```python
from build123d import *

# Parameters (mm, degrees)
SKETCH_W        = 20
SKETCH_H        = 20
PAD_DEPTH       = 6
SKETCH001_R     = 5.5
POCKET_DEPTH    = 3.6
SKETCH002_R     = 3.1
POCKET001_DEPTH = 5
SKETCH003_W     = 5.8
SKETCH003_H     = 5
PAD001_DEPTH    = 6
SKETCH004_W     = 5
SKETCH004_H     = 5.8
PAD002_DEPTH    = 6
SKETCH005_W     = 5.8
SKETCH005_H     = 5
PAD003_DEPTH    = 6
SKETCH006_W     = 5
SKETCH006_H     = 5.8
PAD004_DEPTH    = 6
FILLET_R        = 1.2
FILLET001_R     = 1.2
FILLET002_R     = 1.2
FILLET003_R     = 1.2
FILLET004_R     = 1
FILLET005_R     = 1
FILLET006_R     = 1
FILLET007_R     = 1
FILLET008_R     = 1
FILLET009_R     = 1
FILLET010_R     = 1
FILLET011_R     = 1


with BuildPart() as part:
    # Sketch → Pad (new body)
    with BuildSketch(Plane.XY):
        with Locations((10, 10)):
            Rectangle(SKETCH_W, SKETCH_H)
    extrude(amount=PAD_DEPTH)

    # Sketch001 → Pocket (cut)
    with BuildSketch(Plane.XY.offset(6)):
        with Locations((10, 10)):
            Circle(SKETCH001_R)
    extrude(amount=-POCKET_DEPTH, mode=Mode.SUBTRACT)

    # Sketch002 → Pocket001 (cut)
    with BuildSketch(Plane.XY.offset(2.4)):
        with Locations((10, 10)):
            Circle(SKETCH002_R)
    extrude(amount=-POCKET001_DEPTH, mode=Mode.SUBTRACT)

    # Sketch003 → Pad001 (new body)
    with BuildSketch(Plane(origin=(0, 0, 0), x_dir=(1, 0, 0), z_dir=(0, 0, -1))):
        with Locations((10, -2.5)):
            Rectangle(SKETCH003_W, SKETCH003_H)
    extrude(amount=PAD001_DEPTH)

    # Sketch004 → Pad002 (new body)
    with BuildSketch(Plane(origin=(0, 0, 0), x_dir=(1, 0, 0), z_dir=(0, 0, -1))):
        with Locations((17.5, -10)):
            Rectangle(SKETCH004_W, SKETCH004_H)
    extrude(amount=PAD002_DEPTH)

    # Sketch005 → Pad003 (new body)
    with BuildSketch(Plane(origin=(0, 0, 0), x_dir=(1, 0, 0), z_dir=(0, 0, -1))):
        with Locations((10, -17.5)):
            Rectangle(SKETCH005_W, SKETCH005_H)
    extrude(amount=PAD003_DEPTH)

    # Sketch006 → Pad004 (new body)
    with BuildSketch(Plane(origin=(0, 0, 0), x_dir=(1, 0, 0), z_dir=(0, 0, -1))):
        with Locations((2.5, -10)):
            Rectangle(SKETCH006_W, SKETCH006_H)
    extrude(amount=PAD004_DEPTH)

    # Fillet
    fillet_edges = [part.edges().sort_by_distance(p)[0] for p in [
        (10, 20, 6),
    ]]
    fillet(fillet_edges, radius=FILLET_R)

    # Fillet001
    fillet001_edges = [part.edges().sort_by_distance(p)[0] for p in [
        (10, 0, 6),
    ]]
    fillet(fillet001_edges, radius=FILLET001_R)

    # Fillet002
    fillet002_edges = [part.edges().sort_by_distance(p)[0] for p in [
        (0, 10, 6),
    ]]
    fillet(fillet002_edges, radius=FILLET002_R)

    # Fillet003
    fillet003_edges = [part.edges().sort_by_distance(p)[0] for p in [
        (20, 10, 6),
    ]]
    fillet(fillet003_edges, radius=FILLET003_R)

    # Fillet004
    fillet004_edges = [part.edges().sort_by_distance(p)[0] for p in [
        (15, 10, -6),
    ]]
    fillet(fillet004_edges, radius=FILLET004_R)

    # Fillet005
    fillet005_edges = [part.edges().sort_by_distance(p)[0] for p in [
        (10, 5, -6),
    ]]
    fillet(fillet005_edges, radius=FILLET005_R)

    # Fillet006
    fillet006_edges = [part.edges().sort_by_distance(p)[0] for p in [
        (10, 15, -6),
    ]]
    fillet(fillet006_edges, radius=FILLET006_R)

    # Fillet007
    fillet007_edges = [part.edges().sort_by_distance(p)[0] for p in [
        (5, 10, -6),
    ]]
    fillet(fillet007_edges, radius=FILLET007_R)

    # Fillet008
    fillet008_edges = [part.edges().sort_by_distance(p)[0] for p in [
        (20, 10, -6),
    ]]
    fillet(fillet008_edges, radius=FILLET008_R)

    # Fillet009
    fillet009_edges = [part.edges().sort_by_distance(p)[0] for p in [
        (10, 0, -6),
    ]]
    fillet(fillet009_edges, radius=FILLET009_R)

    # Fillet010
    fillet010_edges = [part.edges().sort_by_distance(p)[0] for p in [
        (10, 20, -6),
    ]]
    fillet(fillet010_edges, radius=FILLET010_R)

    # Fillet011
    fillet011_edges = [part.edges().sort_by_distance(p)[0] for p in [
        (0, 10, -6),
    ]]
    fillet(fillet011_edges, radius=FILLET011_R)


solid = part.part
```
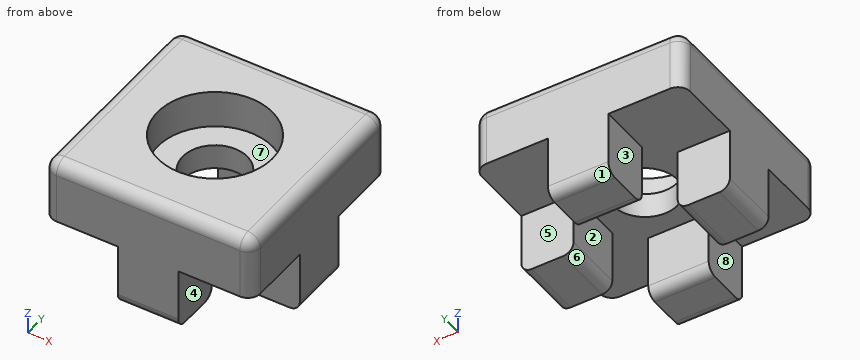
Here's how the part is built. I have some questions about the finished solid (model axes, mm). Face numbers are marked on the shaded views. A direction names the side the tool comes from. Give positions to 0.01 mm unless a question says otherwise; leave off trailing zeros. Order: outer loops, then holes, each group sorted by start corner. A loop starts at its lowest first (then second) coordinate and runs counter-clockwise, first axis right, second up. Notation, with made-up numbers: M -27,-37 L -10,-37 A16 cw -10,-9 Z; hole C -36,24.25 d2. An arc over 180 degrees is marked long. Use a Markdown table: item, result. Add a question column.
1. I need wall thicknesses on probe 1 along Y at (x, z) = (10, 1.3); probe 2 along Y at (x, z) = (10, 3.25); probe 3 along Z at (x, y) = (4.5, 5). Which ranges of each line are inside material? Lowest first, please. Write a range as from..to.
2. On a 3-axis mill with a long thin cutter (end or side, diameter ignored), from which of +Z, -Z, +X, -X, +Y, -Y can I reach the whole of each face in a straight line? I mean the marked faces 4, 5, 6, 7 and 8. Say none if no direction works.
3. Suppose I cut it at B-B (y = 16.25). List the corners of the cut face in (x, z) for me, and give its area (3 significant figures).
4. If we mould it in two halves opening along X, with no side actions, what happens to the marked faces 1, 2 and 3? For each: +X half, -X half, draft (parallel to the pull), parting line (faces both ways), or undercut.
5. Suppose I cut it at C-C (x = 10). List the corners of the cut face in (y, z) for me, and give its area (3 significant figures).
6. Suppose I cut it at D-D (z = -2.25). List the corners of the cut face in (x, y) for me.
7. Suppose I cut it at A-A (z = 4.25). List the corners of the cut face in (x, y) for me.
8. For pin 1 Ø1.5 at (y, z) = (16.5, -1.5) entering from -X; pin 2 Ø1.5 at (x, z) = (16.5, -3.5) entering from -Y; pin 3 Ø1.5 at (y, z) = (3, -2) entering from +X, each with a flat end and sliding along its axis, tell me the tip position at first contact or that it passes through.
Results list:
| question | item | result |
|---|---|---|
| 1 | probe 1 | y = 0..6.9, 13.1..20 |
| 1 | probe 2 | y = 0..4.5, 15.5..20 |
| 1 | probe 3 | z = 0..6 |
| 2 | face 4 | -Z, +X, +Y, -Y |
| 2 | face 5 | -Z, +X, -X, +Y |
| 2 | face 6 | -Z, +Y, -Y |
| 2 | face 7 | +Z |
| 2 | face 8 | -Z, -X, +Y, -Y |
| 3 | outline | M 0,0 L 7.1,0 L 7.1,-6 L 12.9,-6 L 12.9,0 L 20,0 L 20,4.8 A1.2 ccw 18.8,6 L 1.2,6 A1.2 ccw 0,4.8 Z |
| 3 | area | 154 mm² |
| 4 | face 1 | draft |
| 4 | face 2 | undercut |
| 4 | face 3 | -X half |
| 5 | outline | M 0,-5 A1 ccw 1,-6 L 4,-6 A1 ccw 5,-5 L 5,0 L 6.9,0 L 6.9,2.4 L 4.5,2.4 L 4.5,6 L 1.2,6 A1.2 ccw 0,4.8 Z; M 13.1,0 L 15,0 L 15,-5 A1 ccw 16,-6 L 19,-6 A1 ccw 20,-5 L 20,4.8 A1.2 ccw 18.8,6 L 15.5,6 L 15.5,2.4 L 13.1,2.4 Z |
| 5 | area | 124 mm² |
| 6 | outline | M 0,7.1 L 5,7.1 L 5,12.9 L 0,12.9 Z; M 7.1,0 L 12.9,0 L 12.9,5 L 7.1,5 Z; M 7.1,15 L 12.9,15 L 12.9,20 L 7.1,20 Z; M 15,7.1 L 20,7.1 L 20,12.9 L 15,12.9 Z |
| 7 | outline | M 0,1.2 A1.2 ccw 1.2,0 L 18.8,0 A1.2 ccw 20,1.2 L 20,18.8 A1.2 ccw 18.8,20 L 1.2,20 A1.2 ccw 0,18.8 Z; hole C 10,10 d11 |
| 8 | pin 1 | stops at x = 7.1 |
| 8 | pin 2 | stops at y = 7.1 |
| 8 | pin 3 | stops at x = 12.9 |
